Build history of the part. All positions in model axes, mm. A direction names the side the tool comes from. Coordinates: 2 decimals unless noted, no trailing zeros. Loops run counter-clockwise (first coordinate to the right, second up) from the corner with the lowest first, then second, coordinate; pieces in that order, holes last. Notation, with made-up numbers: (7, 50.25) -> (41, 50.25) arc R15 ccw to (41, 79.25) -> close; hole circle Ø11 at (81.5, 56.25). An arc over 180 degrees is marked (long way). One line per item, written item: value. Start each with the question number.
```python
from build123d import *

# Parameters (mm, degrees)
SKETCH_1_R      = 42
SKETCH_1_R_2    = 1.65
SKETCH_1_R_3    = 3
SKETCH_1_W      = 21
SKETCH_1_H      = 21
EXTRUDE_1_DEPTH = 3


with BuildPart() as part:
    # 草图1 → 凸台-拉伸1 (new body)
    with BuildSketch(Plane.XY):
        Circle(SKETCH_1_R)
        with Locations((14.938938215, 8.625)):
            Circle(SKETCH_1_R_2, mode=Mode.SUBTRACT)
        with Locations((14.938938215, -8.625)):
            Circle(SKETCH_1_R_2, mode=Mode.SUBTRACT)
        with Locations((-14.938938215, -8.625)):
            Circle(SKETCH_1_R_2, mode=Mode.SUBTRACT)
        with Locations((-14.938938215, 8.625)):
            Circle(SKETCH_1_R_2, mode=Mode.SUBTRACT)
        with Locations((2.5, 33.5)):
            Circle(SKETCH_1_R_3, mode=Mode.SUBTRACT)
        with Locations((-2.5, 21.5)):
            Circle(SKETCH_1_R_3, mode=Mode.SUBTRACT)
        with Locations(Location((-2.5, -21.5, 0), (0, 0, 180))):
            Circle(SKETCH_1_R_3, mode=Mode.SUBTRACT)
        with Locations(Location((2.5, -33.5, 0), (0, 0, 180))):
            Circle(SKETCH_1_R_3, mode=Mode.SUBTRACT)
        Rectangle(SKETCH_1_W, SKETCH_1_H, mode=Mode.SUBTRACT)
    extrude(amount=EXTRUDE_1_DEPTH)


solid = part.part
```
Item 1: Band-saw the part on C-C, the plane y = -33.5. List the corners of the cut face in (x, z).
Item 2: Band-saw the part on B-B, the plane z = 1.25. Count the separate pieces of the cut face and the enclosed holes in it, and give its area (3 significant figures).
Item 3: Two-plate mould, pull along Y, no slides. Class faces 1 (the face through (-1, -18, 3)), 2 (the face through (40.06, 12.62, 1.48)), 3 (the face through (0, -10.5, 1)): +Y half, -Y half, draft (parallel to the pull), parting line (faces both ways), or undercut.
Item 4: Band-saw the part on A-A, the plane x = 1.5. List the corners of the cut face in (y, z).
Item 5: Band-saw the part on D-D, the plane x = -8. List the corners of the cut face in (y, z).
Item 6: Tool access for faces 4 (the face through (0, 10.5, 1)), 5 (the face through (-1, -18, 0)): list every direction of +Z, -Z, +X, -X, +Y, -Y with a clear straight run to the whole face (end or side of a thin tool).
Item 7: Probe probe 1 along Y at (x, z) = (2.5, 0.3); probe 2 along Y at (x, z) = (-2.5, 1.6); probe 3 along Y at (x, z) = (15, 1.1). List the from-to ranges inside material, lowest first.
Item 8: Drop flat-ended pins along their axis: pin 1 Ø1 at (x, z) = (-2.5, 2) entering from +Y; pin 2 Ø5.5 at (x, y) = (-14.94, -8.62) entering from -Z; pin 3 Ø3 at (x, y) = (14.94, -8.62) entering from -Z; pin 4 Ø0.9 at (x, z) = (4.5, 2) entering from +Y. Give the stop position or say it passes through.
Worked out:
1. outline: (-25.33, 0) -> (-0.5, 0) -> (-0.5, 3) -> (-25.33, 3) -> close; (5.5, 0) -> (25.33, 0) -> (25.33, 3) -> (5.5, 3) -> close
2. separate pieces: 1
2. enclosed holes: 9
2. area: 4,950 mm²
3. face 1: draft
3. face 2: parting line
3. face 3: undercut
4. outline: (-41.97, 0) -> (-36.33, 0) -> (-36.33, 3) -> (-41.97, 3) -> close; (-30.67, 0) -> (-10.5, 0) -> (-10.5, 3) -> (-30.67, 3) -> close; (10.5, 0) -> (30.67, 0) -> (30.67, 3) -> (10.5, 3) -> close; (36.33, 0) -> (41.97, 0) -> (41.97, 3) -> (36.33, 3) -> close
5. outline: (-41.23, 0) -> (-10.5, 0) -> (-10.5, 3) -> (-41.23, 3) -> close; (10.5, 0) -> (41.23, 0) -> (41.23, 3) -> (10.5, 3) -> close
6. face 4: +Z, -Z
6. face 5: -Z, +X, -X, +Y, -Y
7. probe 1: y = -41.93 to -36.5, -30.5 to -10.5, 10.5 to 30.5, 36.5 to 41.93
7. probe 2: y = -41.93 to -24.5, -18.5 to -10.5, 10.5 to 18.5, 24.5 to 41.93
7. probe 3: y = -39.23 to -10.27, -6.98 to 6.98, 10.27 to 39.23
8. pin 1: stops at y = 41.95
8. pin 2: stops at z = 0
8. pin 3: passes through
8. pin 4: stops at y = 41.8
